Design review of the part built by this model. Coordinates are the model's own, in mm. Face numbers are marked on the shaded views. Coordinates: 2 decimals unless noted, no trailing zeros. Order: outer loops, then holes, each group sorted by start corner. A loop starts at its lowest first (then second) coordinate and runs counter-clockwise, first axis right, second up. Notation, with made-up numbers: M -36,75.25 L -21,75.25 A10 cw -21,93.25 Z; hole C -35,54 d8. An arc over 180 degrees is marked long. Answer in a Markdown table with one row per item.
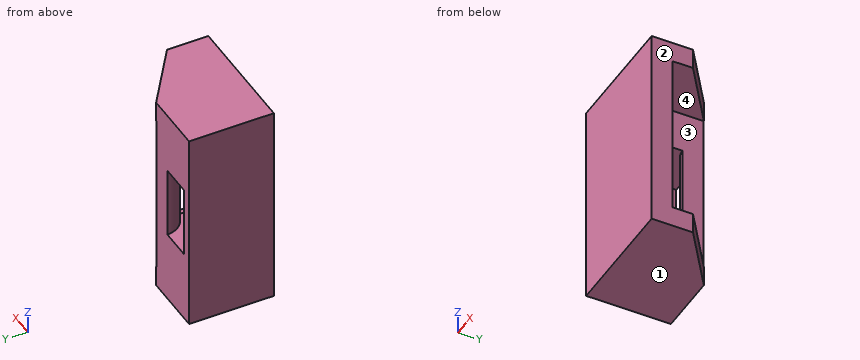
from build123d import *

# Parameters (mm, degrees)
BOSS_EXTRUDE1_DEPTH = 50
SKETCH4_W           = 40
SKETCH4_H           = 15.522388441
CUT_EXTRUDE1_DEPTH  = 15
SKETCH5_W           = 7.5
SKETCH5_H           = 17.5


with BuildPart() as part:
    # Sketch1 → Boss-Extrude1 (new body)
    with BuildSketch(Plane.XY):
        Polygon((0, 0), (0, 20.522388441), (15, 20.522388441), (29.885137085, 10), (29.885137085, 0), align=None)
    extrude(amount=BOSS_EXTRUDE1_DEPTH)

    # Sketch4 → Cut-Extrude1 (cut)
    with BuildSketch(Plane(origin=(29.885137085, 0, 0), x_dir=(0, 0, -1), z_dir=(1, 0, 0))):
        with Locations((-25, 12.761194221)):
            Rectangle(SKETCH4_W, SKETCH4_H)
    extrude(amount=-CUT_EXTRUDE1_DEPTH, mode=Mode.SUBTRACT)

    # Sketch5 → Cut-Revolve1 (revolve, cut)
    with BuildSketch(Plane(origin=(0, 20.522388441, 0), x_dir=(1, 0, 0), z_dir=(0, 1, 0))):
        with Locations((6.135137085, -26.25)):
            Rectangle(SKETCH5_W, SKETCH5_H)
    revolve(axis=Axis((15, 20.522388441, 50), (0, 0, -1)), mode=Mode.SUBTRACT)


solid = part.part
(1) Draft analysis for pull direction Z (two halves, no side actions). For the marked faces 1, 2, 3 and 4, state which applies: pulls with the +Z half, pulls with the -Z half, needs draft (parallel to the pull), parting line crosses it, or undercut.
Return value:
| item | result |
|---|---|
| face 1 | pulls with the -Z half |
| face 2 | needs draft |
| face 3 | undercut |
| face 4 | undercut |
(2) Add section D-D, the plane z = 44. Give the boundary of the cut face in (x, y), and give its area (3 significant figures).
Return value:
| item | result |
|---|---|
| outline | M 0,0 L 29.89,0 L 29.89,5 L 14.89,5 L 14.89,20.52 L 0,20.52 Z |
| area | 380 mm2 |
(3) Add section A-A, the plane z = 24.5. Give the boundary of the cut face in (x, y).
Return value:
| item | result |
|---|---|
| outline | M 0,0 L 29.89,0 L 29.89,5 L 14.89,5 L 14.89,7.91 A12.61 cw 2.39,20.52 L 0,20.52 Z; M 9.89,20.52 A5.11 ccw 14.89,15.41 L 14.89,20.52 Z |
(4) Insertion check: pin 1 Ø8 at (y, z) = (16, 22) entering from +X; pin 2 Ø10 at (x, z) = (21.5, 30.5) entering from +Y. Each pin has a flat end and moves straight along its axis. Give the tip position at first contact, or say it passes through.
Return value:
| item | result |
|---|---|
| pin 1 | stops at x = 14.89 |
| pin 2 | stops at y = 5 |
(5) Add section B-B, the plane y = 16.5. Give the boundary of the cut face in (x, z).
Return value:
| item | result |
|---|---|
| outline | M 0,0 L 20.69,0 L 20.69,5 L 14.89,5 L 14.89,45 L 20.69,45 L 20.69,50 L 0,50 Z; hole M 3.04,17.5 L 11.84,17.5 L 11.84,35 L 3.04,35 Z |
(6) Add section C-C, the plane x = 10.5. Give the boundary of the cut face in (y, z).
Return value:
| item | result |
|---|---|
| outline | M 0,0 L 20.52,0 L 20.52,50 L 0,50 Z; hole M 8.74,17.5 L 18.09,17.5 L 18.09,35 L 8.74,35 Z |
(7) For line 1 along Z through (x, y) = (20.25, 12.25); line 2 along Z through (x, y) = (9, 14.75); line 3 along X through (y, z) = (12.25, 40), list the stretches that pass through material, from the lowest coordinate up. Write a range as from..to.
Return value:
| item | result |
|---|---|
| line 1 | z = 0..5, 45..50 |
| line 2 | z = 0..17.5, 35..50 |
| line 3 | x = 0..14.89 |
